from build123d import *

# Parameters (mm, degrees)
F0_R        = 3
F0_R_2      = 1.5
F1_DEPTH    = 4.5
F2_R        = 20
F3_R        = 25
F4_R        = 25
F5_T1_DEPTH = 24.5
F5_T3_DEPTH = 21.8205080757
F6_R        = 2
F8_DEPTH    = 50
F9_R        = 2
F10_R       = 4


# Not quite as in the source:
# - a fillet or chamfer that OpenCascade refuses, or shapes differently, is made with other operations: its cross-section is extruded or revolved along the edge and cut away or added
# - a feature names something its author has since deleted; it is built from what else it names


with BuildPart() as f1:
    # F0 (on Front) → F1 (new body)
    with BuildSketch(Plane.XZ):
        Polygon((-4, 27), (-4, -4), (4, -4), (4, 4), (2, 4), (2, 27), align=None)
        Circle(F0_R, mode=Mode.SUBTRACT)
        Polygon((-4, 34), (-4, 27), (2, 27), (4, 27), (39.4644660941, 27), (52.3535533906, 14.1109127035), (55.8890872965, 17.6464466094), (39.5355339059, 34), align=None)
        with BuildLine():
            ThreePointArc((25.7442084075, 30.8023647132), (26.3023647132, 28.7557915925), (24.2557915925, 28.1976352868))
            Line((24.2557915925, 28.1976352868), (20.7557915925, 30.1976352868))
            ThreePointArc((20.7557915925, 30.1976352868), (20.1976352868, 32.2442084075), (22.2442084075, 32.8023647132))
            Line((22.2442084075, 32.8023647132), (25.7442084075, 30.8023647132))
        make_face(mode=Mode.SUBTRACT)
        with Locations((52, 18)):
            Circle(F0_R_2, mode=Mode.SUBTRACT)
    extrude(amount=F1_DEPTH)

    # F2
    f2_edges = [f1.edges().sort_by_distance(p)[0] for p in [
        (39.464466, -2.25, 27),
        (2, -2.25, 27),
    ]]
    fillet(f2_edges, radius=F2_R)

    # F3
    f3_edges = [f1.edges().sort_by_distance(p)[0] for p in [
        (-4, -2.25, 34),
    ]]
    fillet(f3_edges, radius=F3_R)

    # F4
    f4_edges = [f1.edges().sort_by_distance(p)[0] for p in [
        (39.535534, -2.25, 34),
    ]]
    fillet(f4_edges, radius=F4_R)

    # F5: fillet of radius 4 on 3 edges, made by hand

    # F5_s2 → F5_t1 (cut)
    with BuildSketch(Plane.XZ.offset(-10)):
        with BuildLine():
            ThreePointArc((0, -4), (2.8284271247, -2.8284271247), (4, 0))
            Line((4, 0), (4, -4))
            Line((4, -4), (0, -4))
        make_face()
        with BuildLine():
            ThreePointArc((-4, 0), (-2.8284271247, -2.8284271247), (0, -4))
            Line((0, -4), (-4, -4))
            Line((-4, -4), (-4, 0))
        make_face()
    extrude(amount=F5_T1_DEPTH, mode=Mode.SUBTRACT)

    # F5_s4 → F5_t3 (cut)
    with BuildSketch(Plane.XZ.offset(-8.6602540378)):
        with BuildLine():
            ThreePointArc((4, 0.5358983849), (3.4641016151, 2.5358983849), (2, 4))
            Line((2, 4), (4, 4))
            Line((4, 4), (4, 0.5358983849))
        make_face()
    extrude(amount=F5_T3_DEPTH, mode=Mode.SUBTRACT)

    # F6
    f6_edges = [f1.edges().sort_by_distance(p)[0] for p in [
        (2, -2.25, 4),
        (52.353553, -2.25, 14.110913),
        (55.889087, -2.25, 17.646447),
    ]]
    fillet(f6_edges, radius=F6_R)

    # F7 (on Top) → F8 (cut, symmetric)
    with BuildSketch(Plane.XY):
        Polygon((34.1801948466, 1.5), (-25.8198051534, 1.5), (-25.8198051534, -2.5), (30.1801948466, -2.5), align=None)
        Polygon((33.5086219714, -2), (29.5086219714, -6), (69.5086219714, -6), (69.5086219714, -2), align=None)
    extrude(amount=F8_DEPTH, both=True, mode=Mode.SUBTRACT)

    # F9
    f9_edges = [f1.edges().sort_by_distance(p)[0] for p in [
        (33.508622, -2, 30.243221),
        (30.180195, -2.5, 30.489996),
    ]]
    fillet(f9_edges, radius=F9_R)

    # F10
    f10_edges = [f1.edges().sort_by_distance(p)[0] for p in [
        (31.008622, -4.5, 30.466524),
        (32.680195, 0, 30.348729),
    ]]
    fillet(f10_edges, radius=F10_R)


solid = f1.part
Part model, mm, in its own coordinate system. A direction names the side the tool comes from. Give positions to 0.01 mm unless a question says otherwise; leave off trailing zeros. Order: outer loops, then holes, each group sorted by start corner. A loop starts at its lowest first (then second) coordinate and runs counter-clockwise, first axis right, second up. Notation, with made-up numbers: (89, 79) -> (124, 79) arc R19 cw to (124, 93) -> close; hole circle Ø8 at (55, -14.5). An arc over 180 degrees is marked (long way). Use one line per item in the form item = value.
(1) Pull direction X, two halves, no side cores. Call faces 1 (the face through (44, 0, 26)), 2 (the face through (-4, -3, 5)), 3 (the face through (26.318, -3.486, 28.785)): +X half, -X half, draft (parallel to the pull), parting line (faces both ways), or undercut.
Solution:
face_1 = draft
face_2 = -X half
face_3 = undercut
(2) Saw through at C-C (z = 31.5). Write the cut outline in (x, y).
Solution:
outline = (10.1, -4.5) -> (20, -4.5) -> (20, -2.5) -> (10.1, -2.5) -> close; (24.52, -4.5) -> (29.35, -4.5) arc R4 ccw to (32.18, -3.33) -> (32.92, -2.59) arc R2 cw to (34.34, -2) -> (40.08, -2) -> (40.08, 0) -> (34.34, 0) arc R4 ccw to (31.51, -1.17) -> (30.77, -1.91) arc R2 cw to (29.35, -2.5) -> (24.52, -2.5) -> close
(3) Flat gauge pins, fed straight in: P1, Ø0.6, axis at y = -4, z = 6, coming from the +X side; P2, Ø9.5, axis at x = 44, z = 25, coming from the -Y side; P3, Ø2.5, axis at x = 27.5, y = -3.5, coming from the -Z side. Where does each tip first touch, or does it go through?
Solution:
P1 = 2
P2 = -2
P3 = 27
(4) Drill centre lines: line 1 (X direction, y = -3.9, z = 0); line 2 (X direction, y = -3.3, z = 5); line 3 (Z direction, x = 52, y = -1.1). Where is each one in solid material? Low to high. Write a range as from..to.
Solution:
line_1 = -4..-3, 3..4
line_2 = -4..2
line_3 = 14.97..16.5, 19.5..21.54
(5) Saw through at D-D (x = 25). Write the cut outline in (y, z), then the cut area to 3 significant figures.
Solution:
outline = (-4.5, 27) -> (-2.5, 27) -> (-2.5, 28) -> (-4.5, 28) -> close; (-4.5, 31.23) -> (-2.5, 31.23) -> (-2.5, 34) -> (-4.5, 34) -> close
area = 7.54 mm²
(6) Saw through at B-B (z = 18). Write the cut outline in (x, y), then the cut area to 3 significant figures.
Solution:
outline = (-2.32, -4.5) -> (5.3, -4.5) -> (5.3, -2.5) -> (-2.32, -2.5) -> close; (48.46, -2) -> (50.5, -2) -> (50.5, 0) -> (48.46, 0) -> close; (53.5, -2) -> (55.03, -2) -> (55.03, 0) -> (53.5, 0) -> close
area = 22.4 mm²
(7) Tool access for faces 4 (the face through (2.17, -3.51, 4.2)), 5 (the face through (25, -3, 34)), 6 (the face through (32.79, -0.31, 30.27)), 7 (the face through (24, -3.5, 31.8)), 8 (the face through (44, -2, 26)): list every direction of +Z, -Z, +X, -X, +Y, -Y with a clear straight run to the whole face (end or side of a thin tool).
Solution:
face_4 = +X, +Y, -Y
face_5 = +Z, +X, -X, +Y, -Y
face_6 = +Z, -Z, -X, +Y
face_7 = +Y, -Y
face_8 = +Z, -Z, +X, -Y
(8) Saw through at A-A (x = 52). Write the cut outline in (y, z), then the cut area to 3 significant figures.
Solution:
outline = (-2, 14.97) -> (0, 14.97) -> (0, 16.5) -> (-2, 16.5) -> close; (-2, 19.5) -> (0, 19.5) -> (0, 21.54) -> (-2, 21.54) -> close
area = 7.13 mm²
